from build123d import *

# Parameters (mm, degrees)
SKETCH_1_W          = 30
SKETCH_1_H          = 24
EXTRUDE_1_DEPTH     = 2
SKETCH_2_W          = 19.5
SKETCH_2_H          = 2
SKETCH_2_W_2        = 2
SKETCH_2_H_2        = 0.5
SKETCH_2_H_3        = 12
EXTRUDE_2_DEPTH     = 5.5
SKETCH_3_W          = 19.5
SKETCH_3_H          = 2
SKETCH_3_W_2        = 2
SKETCH_3_H_2        = 0.5
EXTRUDE_3_DEPTH     = 3
SKETCH_4_W          = 8.5
SKETCH_4_H          = 13
EXTRUDE_4_DEPTH     = 2
SKETCH_5_W          = 8.5
SKETCH_5_H          = 1
EXTRUDE_5_DEPTH     = 8.5
SKETCH_6_W          = 8
SKETCH_6_H          = 7
SKETCH_6_R          = 2.4
EXTRUDE_6_DEPTH     = 2
SKETCH_7_W          = 3.25
SKETCH_7_H          = 3
CUT_EXTRUDE_1_DEPTH = 5.5


with BuildPart() as part:
    # 草图1 → 凸台-拉伸1 (new body)
    with BuildSketch(Plane(origin=(0, 0, 0), x_dir=(1, 0, 0), z_dir=(0, 1, 0))):
        Rectangle(SKETCH_1_W, SKETCH_1_H)
    extrude(amount=EXTRUDE_1_DEPTH)

    # 草图2 → 凸台-拉伸2 (add)
    with BuildSketch(Plane.XZ):
        Polygon((-9.75, 12), (-15, 12), (-15, 6), (-13, 6), (-9.75, 6), (-9.75, 10), align=None)
        with Locations((0, 11)):
            Rectangle(SKETCH_2_W, SKETCH_2_H)
        Polygon((15, 12), (9.75, 12), (9.75, 10), (9.75, 6), (13, 6), (15, 6), align=None)
        with Locations((14, 5.75)):
            Rectangle(SKETCH_2_W_2, SKETCH_2_H_2)
        with Locations((14, -5.75)):
            Rectangle(SKETCH_2_W_2, SKETCH_2_H_2)
        Polygon((9.75, -10), (9.75, -12), (15, -12), (15, -6), (13, -6), (9.75, -6), align=None)
        with Locations((0, -11)):
            Rectangle(SKETCH_2_W, SKETCH_2_H)
        Polygon((-13, -6), (-15, -6), (-15, -12), (-9.75, -12), (-9.75, -10), (-9.75, -6), align=None)
        with Locations((-14, 0)):
            Rectangle(SKETCH_2_W_2, SKETCH_2_H_3)
    extrude(amount=EXTRUDE_2_DEPTH)

    # 草图3 → 凸台-拉伸3 (add)
    with BuildSketch(Plane.XZ.offset(5.5)):
        with Locations((0, 11)):
            Rectangle(SKETCH_3_W, SKETCH_3_H)
        with Locations((0, -11)):
            Rectangle(SKETCH_3_W, SKETCH_3_H)
        with Locations((14, -5.75)):
            Rectangle(SKETCH_3_W_2, SKETCH_3_H_2)
        with Locations((14, 5.75)):
            Rectangle(SKETCH_3_W_2, SKETCH_3_H_2)
    extrude(amount=EXTRUDE_3_DEPTH)

    # 草图4 → 凸台-拉伸4 (add)
    with BuildSketch(Plane(origin=(0, 2, 0), x_dir=(1, 0, 0), z_dir=(0, 1, 0))):
        with Locations((19.25, 0)):
            Rectangle(SKETCH_4_W, SKETCH_4_H)
    extrude(amount=-EXTRUDE_4_DEPTH)

    # 草图5 → 凸台-拉伸5 (add)
    with BuildSketch(Plane.XZ):
        with Locations((19.25, 6)):
            Rectangle(SKETCH_5_W, SKETCH_5_H)
        with Locations((19.25, -6)):
            Rectangle(SKETCH_5_W, SKETCH_5_H)
    extrude(amount=EXTRUDE_5_DEPTH)

    # 草图6 → 凸台-拉伸6 (add)
    # profile 1 of 2: a face of its own
    with BuildSketch(Plane.XZ.offset(8.5)):
        with Locations((4, 15.5)):
            Rectangle(SKETCH_6_W, SKETCH_6_H)
        with Locations(Location((4, 15, 0), (0, 0, 270))):
            Circle(SKETCH_6_R, mode=Mode.SUBTRACT)
    # profile 2 of 2: a face of its own
    with BuildSketch(Plane.XZ.offset(8.5)):
        with Locations((4, -15.5)):
            Rectangle(SKETCH_6_W, SKETCH_6_H)
        with Locations(Location((4, -15, 0), (0, 0, 90))):
            Circle(SKETCH_6_R, mode=Mode.SUBTRACT)
    extrude(amount=-EXTRUDE_6_DEPTH)

    # 草图7 → 切除-拉伸1 (cut)
    with BuildSketch(Plane.XZ.offset(5.5)):
        with Locations((-11.375, 7.5)):
            Rectangle(SKETCH_7_W, SKETCH_7_H)
    extrude(amount=-CUT_EXTRUDE_1_DEPTH, mode=Mode.SUBTRACT)


solid = part.part
Work out the finished part from the listing and answer in its coordinate system (mm). A direction names the side the tool comes from. Give positions to 0.01 mm unless a question says otherwise; leave off trailing zeros. Loops run counter-clockwise (first coordinate to the right, second up) from the corner with the lowest first, then second, coordinate; pieces in that order, holes last. Notation, with made-up numbers: (42, 42) -> (80, 42) arc R32 ccw to (80, 76) -> close; hole circle Ø9 at (57.25, 80). An arc over 180 degrees is marked (long way). Use a Markdown table: item, result. Add a question column.
1) Each of these flat-tipped pins is pushed along its axis until it touches: P1, Ø1, axis at y = -7, z = 6, coming from the -X side; P2, Ø1.6, axis at y = -7, z = 11, coming from the +X side; P3, Ø1, axis at x = 10.5, y = -2.5, coming from the +Z side. Where does it stop, or does it pass through?
2) The part is cut by section A-A, the plane z = 15. Determine the outline of the cut face in (x, y), plus the area to 3 significant figures.
3) The part is cut by section B-B, the plane x = 4. Determine the outline of the cut face in (y, z).
4) For a pull along X with two mould halves and no side action, classify faces 1 (the flat face through (-11, -3, -6)), 2 (the flat face through (15, -2, -9)), 3 (the flat face through (11, -3, 6)), 4 (the flat face through (18, -4, -5.5)) as +X half, -X half, draft (parallel to the pull), parting line (faces both ways), or undercut.
5) Which of the six approach directions +Z, -Z, +X, -X, +Y, -Y give full straight-line access (tool end or side, diameter ignored) to faces 5 (the flat face through (9.75, -3, 8)), 6 (the flat face through (14, -7, 6)), 7 (the flat face through (8, -8, 15))?
6) The part is cut by section D-D, the plane z = -4. Determine the outline of the cut face in (x, y), plus the area to 3 significant figures.
7) The part is cut by section C-C, the plane y = -4.25. Determine the outline of the cut face in (x, z).
8) Consider line 1 along X through (y, z) = (-6.85, -15); line 2 along Z through (x, y) = (-12, -1.75); line 3 along X through (y, z) = (-4.75, -9). Determine where each line is inside the solid, lowest interval first.
Reported:
| question | item | result |
|---|---|---|
| 1 | P1 | stops at x = 13 |
| 1 | P2 | stops at x = 9.75 |
| 1 | P3 | stops at z = 12 |
| 2 | outline | (0, -8.5) -> (1.6, -8.5) -> (1.6, -6.5) -> (0, -6.5) -> close; (6.4, -8.5) -> (8, -8.5) -> (8, -6.5) -> (6.4, -6.5) -> close |
| 2 | area | 6.40 mm^2 |
| 3 | outline | (-8.5, -19) -> (-6.5, -19) -> (-6.5, -17.4) -> (-8.5, -17.4) -> close; (-8.5, -12.6) -> (-6.5, -12.6) -> (-6.5, -12) -> (2, -12) -> (2, 12) -> (-6.5, 12) -> (-6.5, 12.6) -> (-8.5, 12.6) -> (-8.5, 10) -> (0, 10) -> (0, -10) -> (-8.5, -10) -> close; (-8.5, 17.4) -> (-6.5, 17.4) -> (-6.5, 19) -> (-8.5, 19) -> close |
| 4 | face 1 | undercut |
| 4 | face 2 | +X half |
| 4 | face 3 | undercut |
| 4 | face 4 | draft |
| 5 | face 5 | -Y |
| 5 | face 6 | +Z, -X, -Y |
| 5 | face 7 | +Z, +X, +Y, -Y |
| 6 | outline | (-15, -5.5) -> (-13, -5.5) -> (-13, 0) -> (23.5, 0) -> (23.5, 2) -> (-15, 2) -> close |
| 6 | area | 88.0 mm^2 |
| 7 | outline | (-15, -12) -> (15, -12) -> (15, -6.5) -> (23.5, -6.5) -> (23.5, -5.5) -> (13, -5.5) -> (13, -6) -> (9.75, -6) -> (9.75, -10) -> (-9.75, -10) -> (-9.75, -6) -> (-13, -6) -> (-13, 9) -> (-9.75, 9) -> (-9.75, 10) -> (9.75, 10) -> (9.75, 6) -> (13, 6) -> (13, 5.5) -> (23.5, 5.5) -> (23.5, 6.5) -> (15, 6.5) -> (15, 12) -> (-15, 12) -> close |
| 8 | line 1 | x = 0 to 1.6, 6.4 to 8 |
| 8 | line 2 | z = -12 to -6, 9 to 12 |
| 8 | line 3 | x = -15 to -9.75, 9.75 to 15 |
